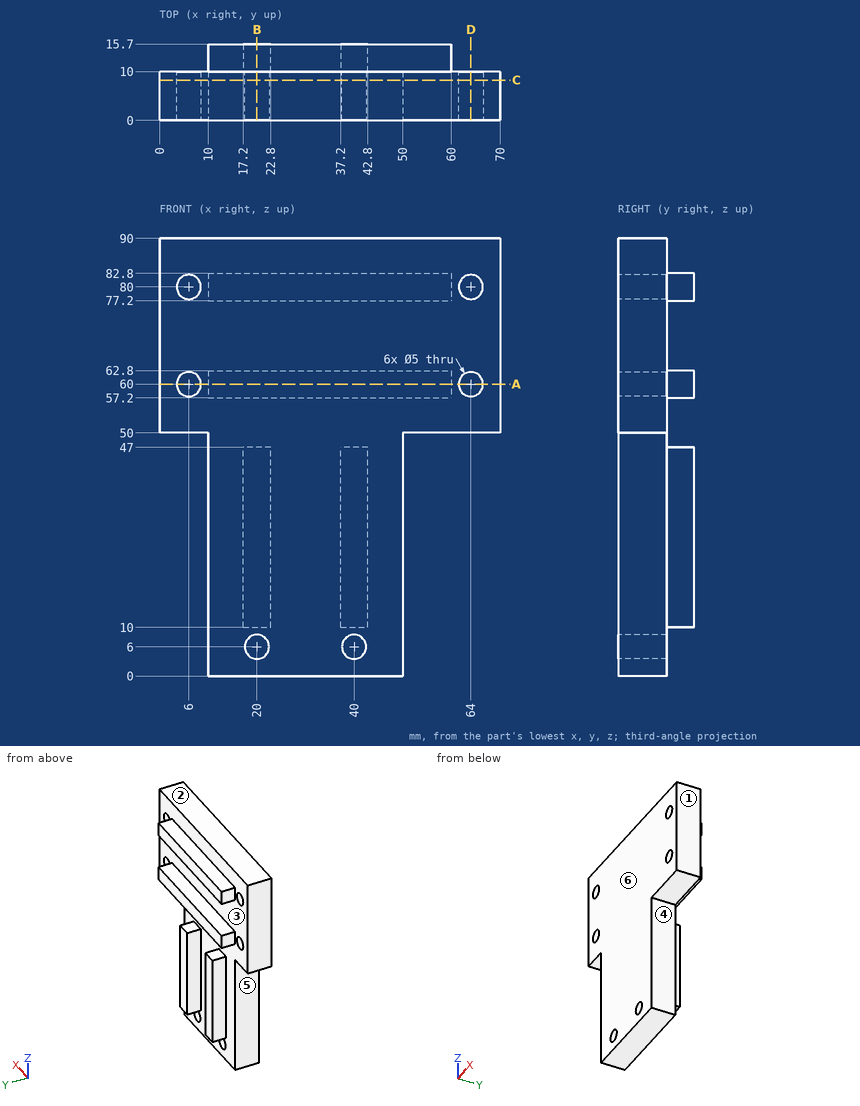
Could you check a few things on this drawing? It's one solid part, dimensions in mm from its lowest x, y, z. A direction names the side the tool comes from. Round coordinates to 2 decimals unless told otherwise and drop trailing zeros. Loops run counter-clockwise (first coordinate to the right, second up) from the corner with the lowest first, then second, coordinate; pieces in that order, holes last. Notation, with made-up numbers: (55, -13) -> (95, -13) arc R32 ccw to (95, 18) -> close; hole circle Ø8 at (83.5, -36.5). An arc over 180 degrees is marked (long way). One line per item, written item: value. Start each with the question number.
1. If we section it at C-C, the plane y = 8.25: Write out the boundary of the cut face in (x, z).
2. If I drill on probe 1 along X at (y, z) = (7, 60); probe 2 along Z at (x, y) = (6, 6); probe 3 along X at (y, z) = (11.25, 17), over which ranges is the centre line in solid material (lowest first)?
3. If we section it at B-B, the plane x = 20: Write out the boundary of the cut face in (y, z).
4. If we mould it in two halves opening along Z, with no side actions, what happens to the marked faces 1, 2 and 3? For each: pulls with the +Z half, pulls with the -Z half, needs draft (parallel to the pull), parting line crosses it, or undercut.
5. For pin 1 (3 mm diameter, centred on y = 13, z = 27, fed in from -X); pin 2 (3 mm diameter, centred on x = 40, y = 14, fed in from +Z); pin 3 (4.5 mm diameter, centred on y = 13, z = 80, fed in from +X), each with a flat end and sliding along its axis, tell me the tip position at first contact or that it passes through.
6. For the marked faces 4, 5 and 6, which set-ups out of +Z, -Z, +X, -X, +Y, -Y let a thin tool reach every point of the face, with its end or its side?
7. If we section it at D-D, the plane x = 64: Write out the boundary of the cut face in (y, z), then the cut area to 3 significant figures.
8. If we section it at A-A, the plane z = 60: Write out the boundary of the cut face in (x, y), then the cut area to 3 significant figures.
Calculated:
1. outline: (0, 50) -> (10, 50) -> (10, 0) -> (50, 0) -> (50, 50) -> (70, 50) -> (70, 90) -> (0, 90) -> close; hole circle Ø5 at (6, 60); hole circle Ø5 at (6, 80); hole circle Ø5 at (20, 6); hole circle Ø5 at (40, 6); hole circle Ø5 at (64, 60); hole circle Ø5 at (64, 80)
2. probe 1: x = 0 to 3.5, 8.5 to 61.5, 66.5 to 70
2. probe 2: z = 50 to 57.5, 62.5 to 77.5, 82.5 to 90
2. probe 3: x = 17.2 to 22.8, 37.2 to 42.8
3. outline: (0, 0) -> (10, 0) -> (10, 3.5) -> (0, 3.5) -> close; (0, 8.5) -> (10, 8.5) -> (10, 10) -> (15.7, 10) -> (15.7, 47) -> (10, 47) -> (10, 57.2) -> (15.7, 57.2) -> (15.7, 62.8) -> (10, 62.8) -> (10, 77.2) -> (15.7, 77.2) -> (15.7, 82.8) -> (10, 82.8) -> (10, 90) -> (0, 90) -> close
4. face 1: needs draft
4. face 2: pulls with the +Z half
4. face 3: undercut
5. pin 1: stops at x = 17.2
5. pin 2: stops at z = 82.8
5. pin 3: stops at x = 60
6. face 4: -Z, +X, +Y, -Y
6. face 5: -Z, -X, +Y, -Y
6. face 6: +Z, -Z, +X, -X, -Y
7. outline: (0, 50) -> (10, 50) -> (10, 57.5) -> (0, 57.5) -> close; (0, 62.5) -> (10, 62.5) -> (10, 77.5) -> (0, 77.5) -> close; (0, 82.5) -> (10, 82.5) -> (10, 90) -> (0, 90) -> close
7. area: 300 mm²
8. outline: (0, 0) -> (3.5, 0) -> (3.5, 10) -> (0, 10) -> close; (8.5, 0) -> (61.5, 0) -> (61.5, 10) -> (60, 10) -> (60, 15.7) -> (10, 15.7) -> (10, 10) -> (8.5, 10) -> close; (66.5, 0) -> (70, 0) -> (70, 10) -> (66.5, 10) -> close
8. area: 885 mm²
